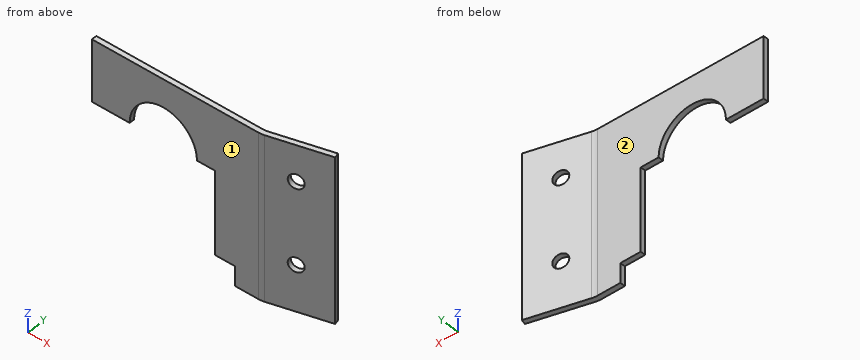
```python
from build123d import *

# Parameters (mm, degrees)
F1_DEPTH      = 60
F1_DEPTH_BACK = 100
F3_DEPTH      = 25
F4_R          = 7
F5_DEPTH      = 25


with BuildPart() as f1:
    # F0 (on Top) → F1 (new body, two sides)
    with BuildSketch(Plane.XY) as f1_sk:
        with BuildLine():
            Line((-70, 0), (-70, -5))
            Line((-70, -5), (93.5252125362, -5))
            ThreePointArc((93.5252125362, -5), (96.1357363806, -4.8288972275), (98.7015934382, -4.3185165258))
            Line((98.7015934382, -4.3185165258), (154.7496448029, 10.6995135747))
            Line((154.7496448029, 10.6995135747), (153.4555495773, 15.5291427062))
            Line((153.4555495773, 15.5291427062), (98.0433309503, 0.6814834742))
            ThreePointArc((98.0433309503, 0.6814834742), (95.4774738927, 0.1711027725), (92.8669500483, 0))
            Line((92.8669500483, 0), (-70, 0))
        make_face()
    extrude(amount=F1_DEPTH)
    extrude(f1_sk.sketch, amount=-F1_DEPTH_BACK)

    # F2 (on Front) → F3 (cut)
    with BuildSketch(Plane.XZ):
        with BuildLine():
            Line((50.5, 0), (33, 0))
            ThreePointArc((33, 0), (0, 33), (-33, 0))
            Line((-33, 0), (-70, 0))
            Line((-70, 0), (-70, -101))
            Line((-70, -101), (70.5, -101))
            Line((70.5, -101), (70.5, -81))
            Line((70.5, -81), (50.5, -81))
            Line((50.5, -81), (50.5, 0))
        make_face()
    extrude(amount=F3_DEPTH, mode=Mode.SUBTRACT)

    # F4 (on face) → F5 (cut)
    with BuildSketch(Plane(origin=(7.6913821948, -28.7046291314, 0), x_dir=(0.9659258263, 0.2588190451, 0), z_dir=(0.2588190451, -0.9659258263, 0))):
        with Locations((120.2459164106, 25)):
            Circle(F4_R)
        with Locations((120.2459164106, -55)):
            Circle(F4_R)
    extrude(amount=-F5_DEPTH, mode=Mode.SUBTRACT)


solid = f1.part
```
Check sheet for the modelled part. Datum: model origin and axes. Units: mm. Face numbers are marked on the shaded views. A direction names the side the tool comes from. Round coordinates to 2 decimals unless told otherwise and drop trailing zeros. Order: outer loops, then holes, each group sorted by start corner. A loop starts at its lowest first (then second) coordinate and runs counter-clockwise, first axis right, second up. Notation, with made-up numbers: M -39.75,31.25 L 8.25,31.25 A26 cw 8.25,60.25 Z; hole C 80,43 d7. An arc over 180 degrees is marked long. Answer in a Markdown table with one row per item.
(1) Gauge pin test, flat ends, axial feed: pin 1 (5 mm diameter, centred on x = -38, y = 2, fed in from +Z); pin 2 (5.5 mm diameter, centred on y = -3.5, z = -93, fed in from -X); pin 3 (2 mm diameter, centred on x = 107.5, z = -24, fed in from +Y); pin 4 (4 mm diameter, centred on x = 60, y = -3, fed in from -Z). Record the tip position at first contact, or that the pin passes through.
Findings:
| item | result |
|---|---|
| pin 1 | stops at z = 60 |
| pin 2 | stops at x = 70.5 |
| pin 3 | stops at y = 3.48 |
| pin 4 | stops at z = -81 |
(2) Section check D-D on x = -42. Record the boundary of the cut face in (y, z), plus the area to 3 significant figures.
Findings:
| item | result |
|---|---|
| outline | M -5,0 L 0,0 L 0,60 L -5,60 Z |
| area | 300 mm^2 |
(3) Section check A-A on z = -42. Record the boundary of the cut face in (x, y).
Findings:
| item | result |
|---|---|
| outline | M 50.5,-5 L 93.53,-5 A20 ccw 98.7,-4.32 L 154.75,10.7 L 153.46,15.53 L 98.04,0.68 A20 cw 92.87,0 L 50.5,0 Z |
(4) Section check B-B on x = 0. Record the boundary of the cut face in (y, z).
Findings:
| item | result |
|---|---|
| outline | M -5,33 L 0,33 L 0,60 L -5,60 Z |
(5) Set-up check for the marked faces 1 and 2: record each of +Z, -Z, +X, -X, +Y, -Y from which the full face is reachable in a straight line by a thin tool's end or side.
Findings:
| item | result |
|---|---|
| face 1 | +Z, -Z, +X, -X, -Y |
| face 2 | +Z, -Z, -X, +Y |
(6) Section check C-C on z = 50.5. Record the boundary of the cut face in (x, y), plus the area to 3 significant figures.
Findings:
| item | result |
|---|---|
| outline | M -70,-5 L 93.53,-5 A20 ccw 98.7,-4.32 L 154.75,10.7 L 153.46,15.53 L 98.04,0.68 A20 cw 92.87,0 L -70,0 Z |
| area | 1,130 mm^2 |
(7) Material ranges on line 1 along Z through (x, y) = (125.5, 7); line 2 along Y through (x, z) = (58, -56); line 3 along Z through (x, y) = (36, -1.25), recorded low to high. Write a range as from..to.
Findings:
| item | result |
|---|---|
| line 1 | z = -100..-61.42, -48.58..18.58, 31.42..60 |
| line 2 | y = -5..0 |
| line 3 | z = 0..60 |
